Check sheet for the modelled part. Datum: model origin and axes. Units: mm. Give positions to 0.01 mm unless a question says otherwise; leave off trailing zeros. Write each loop counter-clockwise with the first axis right and the second up, starting at its lowest first coordinate (ties: lowest second). Pieces come first, ordered by that corner, then holes. Notation, with made-up numbers: (81.5, -11) -> (119.5, -11) arc R22 cw to (119.5, 10) -> close; hole circle Ø11 at (-20, 25.25). An arc over 180 degrees is marked (long way). Use a Markdown table: item, result. Add a question column.
1. Cross-section at A-A (z = 26). Enter the section's corners in (x, y), then the cut area to 3 significant figures.
2. Scan lines: probe 1 along X at (y, z) = (0, 42.75); probe 2 along Y at (x, z) = (-20.5, 26.5); probe 3 along X at (y, z) = (-6.35, 15). Record each from-to range of solid material in increasing order. Write a range as [from, to].
3. Cross-section at B-B (z = 51.5). Enter the section's corners in (x, y), then the cut area to 3 significant figures.
4. Gauge pin test, flat ends, axial feed: P1, Ø3, axis at x = -20.64, y = 6.35, coming from the -Z side; P2, Ø3.5, axis at x = -20.29, y = 0, coming from the +Z side. Record the tip position at first contact, or that the pin passes through.
from build123d import *

# Parameters (mm, degrees)
F0_W     = 31.75
F0_H     = 63.0428
F1_DEPTH = 12.7
F3_D     = 3.4544
F3_DEPTH = 27.78125
F3_TIP   = 1.0378064612
F5_D     = 4.0386
F5_DEPTH = 27.78125
F5_TIP   = 1.213317848


with BuildPart() as f1:
    # F0 (on Front) → F1 (new body, symmetric)
    with BuildSketch(Plane.XZ):
        with Locations((-15.875, 31.5214)):
            Rectangle(F0_W, F0_H)
    extrude(amount=F1_DEPTH, both=True)

    # F3
    with Locations(Plane(origin=(0, 0, 0), x_dir=(1, 0, 0), z_dir=(0, 0, -1))):
        with Locations((-20.6375, 6.35), (-4.7625, 6.35), (-4.7625, -6.35), (-20.6375, -6.35)):
            Hole(F3_D / 2, depth=F3_DEPTH)
            with Locations((0, 0, -(F3_DEPTH + F3_TIP / 2))):  # 118° drill point
                Cone(0, F3_D / 2, F3_TIP, mode=Mode.SUBTRACT)

    # F5
    with Locations(Plane.XY.offset(63.0428)):
        with Locations((-7.5946, 0), (-20.2946, 0)):
            Hole(F5_D / 2, depth=F5_DEPTH)
            with Locations((0, 0, -(F5_DEPTH + F5_TIP / 2))):  # 118° drill point
                Cone(0, F5_D / 2, F5_TIP, mode=Mode.SUBTRACT)


solid = f1.part
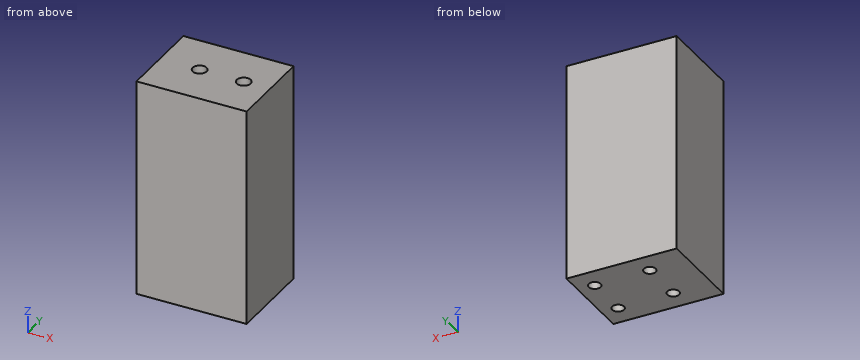
Worked answers:
| question | item | result |
|---|---|---|
| 1 | outline | (-31.75, -12.7) -> (0, -12.7) -> (0, 12.7) -> (-31.75, 12.7) -> close; hole circle Ø3.45 at (-20.64, -6.35); hole circle Ø3.45 at (-20.64, 6.35); hole circle Ø3.45 at (-4.76, -6.35); hole circle Ø3.45 at (-4.76, 6.35) |
| 1 | area | 769 mm² |
| 2 | probe 1 | x = [-31.75, -22.31], [-18.28, -9.61], [-5.58, 0] |
| 2 | probe 2 | y = [-12.7, -8.07], [-4.63, 4.63], [8.07, 12.7] |
| 2 | probe 3 | x = [-31.75, -22.36], [-18.91, -6.49], [-3.04, 0] |
| 3 | outline | (-31.75, -12.7) -> (0, -12.7) -> (0, 12.7) -> (-31.75, 12.7) -> close; hole circle Ø4.04 at (-20.29, 0); hole circle Ø4.04 at (-7.59, 0) |
| 3 | area | 781 mm² |
| 4 | P1 | stops at z = 27.92 |
| 4 | P2 | stops at z = 35.1 |
